```python
from build123d import *

# Parameters (mm, degrees)
SKETCH1_W           = 190
SKETCH1_H           = 70
BOSS_EXTRUDE1_DEPTH = 60
SKETCH2_W           = 178.169104448
SKETCH2_H           = 60
CUT_EXTRUDE1_DEPTH  = 50
FILLET2_R           = 5.08
SKETCH5_R           = 3.5
CUT_EXTRUDE3_DEPTH  = 11.210906631
SKETCH6_W           = 179.69669377
SKETCH6_H           = 60
BOSS_EXTRUDE3_DEPTH = 20
SKETCH7_W           = 15
SKETCH7_H           = 33.02
CUT_EXTRUDE4_DEPTH  = 16.51
SKETCH9_W           = 7
SKETCH9_H           = 5
CUT_EXTRUDE5_DEPTH  = 6.929984537
SKETCH11_W          = 91
SKETCH11_H          = 59
CUT_EXTRUDE6_DEPTH  = 17
SKETCH13_W          = 21.297722751
SKETCH13_H          = 5.714951011
CUT_EXTRUDE7_DEPTH  = 26.645395744
SKETCH16_W          = 73.169104448
SKETCH16_H          = 60
BOSS_EXTRUDE9_DEPTH = 15


with BuildPart() as part:
    # Sketch1 → Boss-Extrude1 (new body)
    with BuildSketch(Plane(origin=(0, 0, 0), x_dir=(1, 0, 0), z_dir=(0, 1, 0))):
        Rectangle(SKETCH1_W, SKETCH1_H)
    extrude(amount=BOSS_EXTRUDE1_DEPTH)

    # Sketch2 → Cut-Extrude1 (cut)
    with BuildSketch(Plane(origin=(0, 60, 0), x_dir=(1, 0, 0), z_dir=(0, 1, 0))):
        Rectangle(SKETCH2_W, SKETCH2_H)
    extrude(amount=-CUT_EXTRUDE1_DEPTH, mode=Mode.SUBTRACT)

    # Fillet2
    fillet2_edges = [part.edges().sort_by_distance(p)[0] for p in [
        (-95, 30, -35),
        (95, 30, -35),
        (95, 30, 35),
        (-95, 30, 35),
    ]]
    fillet(fillet2_edges, radius=FILLET2_R)

    # Sketch5 → Cut-Extrude3 (cut)
    with BuildSketch(Plane(origin=(0, 0, -35), x_dir=(-1, 0, 0), z_dir=(0, 0, -1))):
        with Locations((-49.92, 53)):
            Circle(SKETCH5_R)
    extrude(amount=-CUT_EXTRUDE3_DEPTH, mode=Mode.SUBTRACT)

    # Sketch6 → Boss-Extrude3 (add)
    with BuildSketch(Plane(origin=(0, 10, 0), x_dir=(1, 0, 0), z_dir=(0, 1, 0))):
        with Locations((-0.763794661, 0)):
            Rectangle(SKETCH6_W, SKETCH6_H)
    extrude(amount=BOSS_EXTRUDE3_DEPTH)

    # Sketch7 → Cut-Extrude4 (cut)
    with BuildSketch(Plane.ZY.offset(-89.084552224)):
        with Locations((12.5, 51.51)):
            Rectangle(SKETCH7_W, SKETCH7_H)
    extrude(amount=-CUT_EXTRUDE4_DEPTH, mode=Mode.SUBTRACT)

    # Sketch9 → Cut-Extrude5 (cut)
    with BuildSketch(Plane(origin=(4.741106384, 60, 0), x_dir=(1, 0, 0), z_dir=(0, 1, 0))):
        with Locations((45.208400252, 32.5)):
            Rectangle(SKETCH9_W, SKETCH9_H)
    extrude(amount=-CUT_EXTRUDE5_DEPTH, mode=Mode.SUBTRACT)

    # Sketch11 → Cut-Extrude6 (cut)
    with BuildSketch(Plane.XZ):
        with Locations((-37.248482646, 0)):
            Rectangle(SKETCH11_W, SKETCH11_H)
    extrude(amount=-CUT_EXTRUDE6_DEPTH, mode=Mode.SUBTRACT)

    # Sketch13 → Cut-Extrude7 (cut)
    with BuildSketch(Plane.XZ.offset(-17)):
        with Locations((-2.397344022, 29.141507707)):
            Rectangle(SKETCH13_W, SKETCH13_H)
    extrude(amount=-CUT_EXTRUDE7_DEPTH, mode=Mode.SUBTRACT)

    # Sketch16 → Boss-Extrude9 (add)
    with BuildSketch(Plane(origin=(0, 30, 0), x_dir=(1, 0, 0), z_dir=(0, 1, 0))):
        with Locations((-52.5, 0)):
            Rectangle(SKETCH16_W, SKETCH16_H)
    extrude(amount=BOSS_EXTRUDE9_DEPTH)


solid = part.part
```
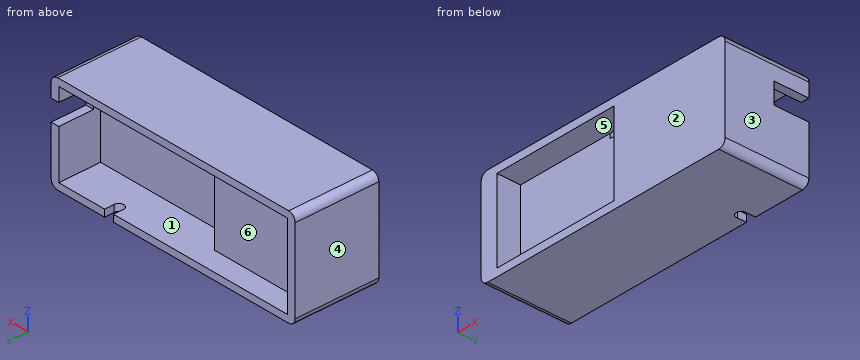
The listing builds one solid part. Answer for the finished solid, in the listing's coordinates (mm). Face numbers are marked on the shaded views. A direction names the side the tool comes from. Coordinates: 2 decimals unless noted, no trailing zeros. Write each loop counter-clockwise with the first axis right and the second up, starting at its lowest first coordinate (ties: lowest second). Pieces come first, ordered by that corner, then holes. Notation, with made-up numbers: (3.25, 79.25) - (25.25, 79.25) arc R27 ccw to (25.25, 102.25) - close; hole circle Ø9 at (16, 11). An arc over 180 degrees is marked (long way). One line per item, written item: value.
1) A tool of negligible diameter and unlimited length cuts with its end or side. For the marked faces 4, 5 and 6, from which of +Z, -Z, +X, -X, +Y, -Y can it reach the whole face along a straight path? Write none if from no direction.
Geometry check:
face 4: +Z, -Z, -X, +Y, -Y
face 5: -Y
face 6: +Y
2) Find section D-D (x = -40.5). Give the vertices of the cut face in (y, z), and give its area (3 significant figures).
Geometry check:
outline: (0, -35) - (60, -35) - (60, -30) - (45, -30) - (45, 30) - (60, 30) - (60, 35) - (0, 35) - (0, 29.5) - (17, 29.5) - (17, -29.5) - (0, -29.5) - close
area: 2,300 mm2
3) Find section A-A (y = 32). Give the vertices of the cut face in (x, z), and give its area (3 significant figures).
Geometry check:
outline: (-95, -29.92) arc R5.08 ccw to (-89.92, -35) - (89.92, -35) arc R5.08 ccw to (95, -29.92) - (95, 29.92) arc R5.08 ccw to (89.92, 35) - (-89.92, 35) arc R5.08 ccw to (-95, 29.92) - close; hole (-15.92, -30) - (89.08, -30) - (89.08, 30) - (8.25, 30) - (8.25, 32) - (-13.05, 32) - (-13.05, 30) - (-15.92, 30) - close
area: 6,940 mm2
4) Each of these flat-tipped pins is pushed along its axis until it touches: pin 1 Ø1.8 at (x, y) = (92, 47) entering from -Z; pin 2 Ø2.5 at (y, z) = (58, -32.5) entering from +X; pin 3 Ø4 at (x, z) = (-13.5, 13.5) entering from -Y; pin 4 Ø5.5 at (y, z) = (57.5, -32) entering from -X. Where does it stop, or does it pass through?
Geometry check:
pin 1: stops at z = -34.86
pin 2: stops at x = 94.82
pin 3: stops at y = 17
pin 4: stops at x = -95
5) Consider line 1 along X through (y, z) = (38, 27); line 2 along X through (y, z) = (15, -27); line 3 along Z through (x, y) = (45, 42). Determine where each line is inside the solid, lowest interval first. Write a range as from..to.
Geometry check:
line 1: x = -95..-15.92, 89.08..95
line 2: x = -95..-82.75, 8.25..95
line 3: z = -35..-30, 30..35
6) For a pull along X with two mould halves and no side action, classify the marked faces 1, 2 and 3 as pulls with the +X half, pulls with the -X half, needs draft (parallel to the pull), parting line crosses it, or undercut.
Geometry check:
face 1: undercut
face 2: needs draft
face 3: pulls with the +X half
7) Find section B-B (x = 2). Give the vertices of the cut face in (y, z), and give its area (3 significant figures).
Geometry check:
outline: (0, -35) - (60, -35) - (60, -30) - (30, -30) - (30, 26.28) - (17, 26.28) - (17, -29.5) - (0, -29.5) - close; (0, 29.5) - (17, 29.5) - (17, 32) - (43.65, 32) - (43.65, 30) - (60, 30) - (60, 35) - (0, 35) - close
area: 1,300 mm2
8) Find section C-C (z = -19). Give the vertices of the cut face in (x, y).
Geometry check:
outline: (-95, 0) - (-82.75, 0) - (-82.75, 17) - (8.25, 17) - (8.25, 0) - (95, 0) - (95, 60) - (89.08, 60) - (89.08, 30) - (-15.92, 30) - (-15.92, 45) - (-89.08, 45) - (-89.08, 60) - (-95, 60) - close
